```python
from build123d import *

# Parameters (mm, degrees)
SKETCH3_W            = 50
SKETCH3_H            = 80
BOSS_EXTRUDE1_DEPTH  = 5
SKETCH5_R            = 6
SKETCH5_R_2          = 3.25
BOSS_EXTRUDE2_DEPTH  = 6
BOSS_EXTRUDE3_DEPTH  = 5
M4_CLEARANCE_HOLE1_D = 4.8
FILLET1_R            = 3


with BuildPart() as part:
    # Sketch3 → Boss-Extrude1 (new body)
    with BuildSketch(Plane.XY):
        Rectangle(SKETCH3_W, SKETCH3_H)
    extrude(amount=BOSS_EXTRUDE1_DEPTH)

    # Sketch5 → Boss-Extrude2 (add)
    # profile 1 of 4: a face of its own
    with BuildSketch(Plane.XY.offset(5)):
        with Locations((-12.434, -28.575)):
            Circle(SKETCH5_R)
        with Locations((-12.434, -28.575)):
            Circle(SKETCH5_R_2, mode=Mode.SUBTRACT)
    # profile 2 of 4: a face of its own
    with BuildSketch(Plane.XY.offset(5)):
        with Locations((18.046, -28.575)):
            Circle(SKETCH5_R)
        with Locations((18.046, -28.575)):
            Circle(SKETCH5_R_2, mode=Mode.SUBTRACT)
    # profile 3 of 4: a face of its own
    with BuildSketch(Plane.XY.offset(5)):
        with Locations((-12.434, 28.575)):
            Circle(SKETCH5_R)
        with Locations((-12.434, 28.575)):
            Circle(SKETCH5_R_2, mode=Mode.SUBTRACT)
    # profile 4 of 4: a face of its own
    with BuildSketch(Plane.XY.offset(5)):
        with Locations((18.046, 28.575)):
            Circle(SKETCH5_R)
        with Locations((18.046, 28.575)):
            Circle(SKETCH5_R_2, mode=Mode.SUBTRACT)
    extrude(amount=BOSS_EXTRUDE2_DEPTH)

    # Sketch8 → Boss-Extrude3 (add)
    with BuildSketch(Plane.XY.offset(5)):
        with BuildLine():
            Line((0, 43), (0, 40))
            Line((0, 40), (7.5, 40))
            Line((7.5, 40), (7.5, 50))
            Line((7.5, 50), (0, 50))
            Line((0, 50), (0, 47))
            ThreePointArc((0, 47), (1.414213562, 46.414213562), (2, 45))
            ThreePointArc((2, 45), (1.414213562, 43.585786438), (0, 43))
        make_face()
        with BuildLine():
            Line((-7.5, 50), (-7.5, 40))
            Line((-7.5, 40), (0, 40))
            Line((0, 40), (0, 43))
            ThreePointArc((0, 43), (-2, 45), (0, 47))
            Line((0, 47), (0, 50))
            Line((0, 50), (-7.5, 50))
        make_face()
        with BuildLine():
            ThreePointArc((0, 47), (-2, 45), (0, 43))
            Line((0, 43), (0, 47))
        make_face()
        with BuildLine():
            Line((0, 47), (0, 43))
            ThreePointArc((0, 43), (1.414213562, 43.585786438), (2, 45))
            ThreePointArc((2, 45), (1.414213562, 46.414213562), (0, 47))
        make_face()
    boss_extrude3 = extrude(amount=-BOSS_EXTRUDE3_DEPTH)

    # M4 Clearance Hole1 (through all)
    with Locations(Plane.XY.offset(5)):
        with Locations((0, 45)):
            m4_clearance_hole1 = Hole(M4_CLEARANCE_HOLE1_D / 2)

    # Mirror1: Boss-Extrude3, M4 Clearance Hole1 across plane
    add(boss_extrude3.mirror(Plane.ZX))
    add(m4_clearance_hole1.mirror(Plane.ZX), mode=Mode.SUBTRACT)

    # Fillet1
    fillet1_edges = [part.edges().sort_by_distance(p)[0] for p in [
        (-7.5, 40, 2.5),
        (-7.5, 50, 2.5),
        (7.5, 50, 2.5),
        (7.5, 40, 2.5),
        (-7.5, -50, 2.5),
        (-7.5, -40, 2.5),
        (7.5, -40, 2.5),
        (7.5, -50, 2.5),
        (25, -40, 2.5),
        (-25, -40, 2.5),
        (-25, 40, 2.5),
        (25, 40, 2.5),
    ]]
    fillet(fillet1_edges, radius=FILLET1_R)


solid = part.part
```
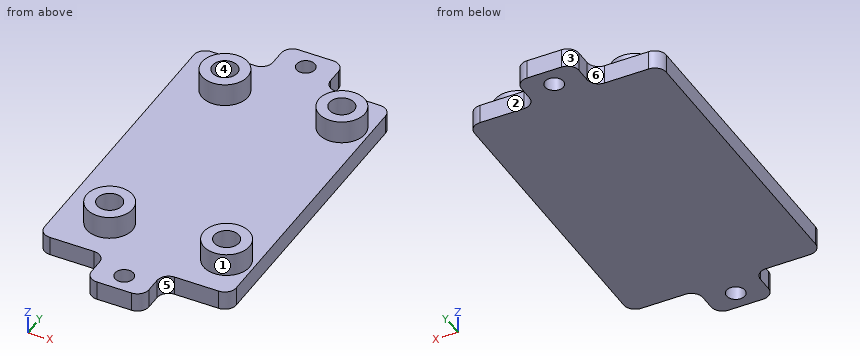
Work out the finished part from the listing and answer in its coordinate system (mm). Face numbers are marked on the shaded views. A direction names the side the tool comes from. Coordinates: 2 decimals unless noted, no trailing zeros. Write each loop counter-clockwise with the first axis right and the second up, starting at its lowest first coordinate (ties: lowest second). Pieces come first, ordered by that corner, then holes.
Q1. A cutting plane is placed at B-B, the plane y = -45. Give the vertices of the cut face in (x, z), then the cut area to 3 significant figures.
Q2. Each of these flat-tipped pins is pushed along its axis until it touches: pin 1 Ø1.5 at (x, y) = (-3.5, 31) entering from -Z; pin 2 Ø1 at (x, z) = (-5.5, 9.5) entering from -Y; pin 3 Ø1.5 at (x, z) = (16, 3.5) entering from +Y; pin 4 Ø2 at (x, y) = (18, 27) entering from +Z. Where does it stop, or does it pass through?
Q3. A cutting plane is placed at C-C, the plane z = 6.75. Give the vertices of the cut face in (x, y) (3 decimals).
Q4. Which of the six approach directions +Z, -Z, +X, -X, +Y, -Y give full straight-line access (tool end or side, diameter ignored) to the marked faces 1, 2 and 3?
Q5. A cutting plane is placed at D-D, the plane x = -17. Give the vertices of the cut face in (y, z).
Q6. Find the intervals of material crossed by line 1 (Y direction, x = 0, z = 2.2); line 2 (X direction, y = 30, z = 6); line 3 (X direction, y = -31, z = 7), in increasing order.
Q7. A cutting plane is placed at A-A, the plane x = 0. Give the vertices of the cut face in (y, z).
Q8. Determine the mould class of the marked faces 4, 5 and 6 for opening direction Y: released by +Y, released by -Y, zero draft, split by the parting line, or undercut.
Findings below:
1. outline: (-7.5, 0) - (-2.4, 0) - (-2.4, 5) - (-7.5, 5) - close; (2.4, 0) - (7.5, 0) - (7.5, 5) - (2.4, 5) - close
1. area: 51.0 mm2
2. pin 1: stops at z = 0
2. pin 2: passes through
2. pin 3: stops at y = 40
2. pin 4: stops at z = 5
3. outline: circle Ø12 at (-12.434, -28.575); circle Ø12 at (-12.434, 28.575); circle Ø12 at (18.046, -28.575); circle Ø12 at (18.046, 28.575); hole circle Ø6.5 at (-12.434, -28.575); hole circle Ø6.5 at (-12.434, 28.575); hole circle Ø6.5 at (18.046, -28.575); hole circle Ø6.5 at (18.046, 28.575)
4. face 1: +Z
4. face 2: +Z, -Z, +X, +Y
4. face 3: +Z, -Z, -X, +Y
5. outline: (-40, 0) - (40, 0) - (40, 5) - (32.47, 5) - (32.47, 11) - (24.68, 11) - (24.68, 5) - (-24.68, 5) - (-24.68, 11) - (-32.47, 11) - (-32.47, 5) - (-40, 5) - close
6. line 1: y = -50 to -47.4, -42.6 to 42.6, 47.4 to 50
6. line 2: x = -18.26 to -15.35, -9.51 to -6.61, 12.22 to 15.13, 20.97 to 23.87
6. line 3: x = -17.92 to -14.6, -10.27 to -6.95, 12.56 to 15.88, 20.21 to 23.53
7. outline: (-50, 0) - (-47.4, 0) - (-47.4, 5) - (-50, 5) - close; (-42.6, 0) - (42.6, 0) - (42.6, 5) - (-42.6, 5) - close; (47.4, 0) - (50, 0) - (50, 5) - (47.4, 5) - close
8. face 4: undercut
8. face 5: released by -Y
8. face 6: released by +Y
